Geometry check sheet. Reference: the model listing, model coordinates, mm. Round coordinates to 2 decimals unless told otherwise and drop trailing zeros. Loops run counter-clockwise (first coordinate to the right, second up) from the corner with the lowest first, then second, coordinate; pieces in that order, holes last. Notation, with made-up numbers: (57, 87.25) - (82, 87.25) arc R22 ccw to (82, 109.25) - close; hole circle Ø5 at (-23.5, 45). An arc over 180 degrees is marked (long way). Answer as CSV lines item,"result". Start each with the question number.
1) Cross-section at D-D on y = 232.7. Record the boundary of the cut face in (x, z).
2) Depth check by flat-ended pin: P1, Ø11.5, axis at x = 100, y = 232.7, coming from the +Z side; P2, Ø18, axis at x = 63, z = -36.5, coming from the +Y side; P3, Ø4, axis at x = 138, y = 216, coming from the -Z side. Enter the tip coordinate at first touch or a pass-through.
3) Cross-section at C-C on z = -30. Record the boundary of the cut face in (x, y), and give its area (3 significant figures).
4) Cross-section at A-A on x = 100. Record the boundary of the cut face in (y, z).
5) Draft check along Y on faces 1 (the flat face through (99, 2.7, -30)), 2 (the cylindrical face through (95.381, 34.615, 1.331)), 3 (the flat face through (99, 157, 0)). Enter one of: released by +Y, released by -Y, zero draft, split by the parting line, or undercut.
6) Thickness scan on line 1 along X through (y, z) = (1, -30); line 2 along Y through (x, z) = (100, 1); line 3 along Z through (x, y) = (165, 1.8). Record the ranges inside material, lowest first.
7) Cross-section at B-B on x = 35. Record the boundary of the cut face in (y, z).
from build123d import *

# Parameters (mm, degrees)
SKETCH1_W           = 200
SKETCH1_H           = 60
SKETCH1_R           = 5
BOSS_EXTRUDE1_DEPTH = 2.7
SKETCH2_W           = 200
SKETCH2_H           = 306.7
SKETCH2_R           = 5
BOSS_EXTRUDE2_DEPTH = 2.7


with BuildPart() as part:
    # Sketch1 → Boss-Extrude1 (new body)
    with BuildSketch(Plane(origin=(0, 0, 0), x_dir=(1, 0, 0), z_dir=(0, 1, 0))):
        with Locations((100, 30)):
            Rectangle(SKETCH1_W, SKETCH1_H)
        with Locations(Location((35, 30, 0), (0, 0, 90))):
            Circle(SKETCH1_R, mode=Mode.SUBTRACT)
        with Locations(Location((165, 30, 0), (0, 0, 90))):
            Circle(SKETCH1_R, mode=Mode.SUBTRACT)
    extrude(amount=BOSS_EXTRUDE1_DEPTH)

    # Sketch2 → Boss-Extrude2 (add)
    with BuildSketch(Plane.XY):
        with Locations((100, 153.35)):
            Rectangle(SKETCH2_W, SKETCH2_H)
        with Locations(Location((100, 32.7, 0), (0, 0, 180))):
            Circle(SKETCH2_R, mode=Mode.SUBTRACT)
        with Locations(Location((100, 232.7, 0), (0, 0, 180))):
            Circle(SKETCH2_R, mode=Mode.SUBTRACT)
    extrude(amount=BOSS_EXTRUDE2_DEPTH)


solid = part.part
Answer block:
1,outline,"(0, 0) - (95, 0) - (95, 2.7) - (0, 2.7) - close; (105, 0) - (200, 0) - (200, 2.7) - (105, 2.7) - close"
2,P1,"stops at z = 2.7"
2,P2,"stops at y = 2.7"
2,P3,"stops at z = 0"
3,outline,"(0, 0) - (30, 0) - (30, 2.7) - (0, 2.7) - close; (40, 0) - (160, 0) - (160, 2.7) - (40, 2.7) - close; (170, 0) - (200, 0) - (200, 2.7) - (170, 2.7) - close"
3,area,"486 mm^2"
4,outline,"(0, -60) - (2.7, -60) - (2.7, 0) - (27.7, 0) - (27.7, 2.7) - (0, 2.7) - close; (37.7, 0) - (227.7, 0) - (227.7, 2.7) - (37.7, 2.7) - close; (237.7, 0) - (306.7, 0) - (306.7, 2.7) - (237.7, 2.7) - close"
5,face 1,"released by +Y"
5,face 2,"undercut"
5,face 3,"zero draft"
6,line 1,"x = 0 to 30, 40 to 160, 170 to 200"
6,line 2,"y = 0 to 27.7, 37.7 to 227.7, 237.7 to 306.7"
6,line 3,"z = -60 to -35, -25 to 2.7"
7,outline,"(0, -60) - (2.7, -60) - (2.7, -35) - (0, -35) - close; (0, -25) - (2.7, -25) - (2.7, 0) - (306.7, 0) - (306.7, 2.7) - (0, 2.7) - close"
